Part model, mm, in its own coordinate system. A direction names the side the tool comes from. Give positions to 0.01 mm unless a question says otherwise; leave off trailing zeros. Write each loop counter-clockwise with the first axis right and the second up, starting at its lowest first coordinate (ties: lowest second). Pieces come first, ordered by that corner, then holes.
from build123d import *

# Parameters (mm, degrees)
SKETCH1_R           = 1.5
BOSS_EXTRUDE1_DEPTH = 2
SKETCH3_OUTSIDE_W   = 31.914
SKETCH3_OUTSIDE_H   = 31.796
SKETCH3_OUTSIDE_R   = 11.40725
CUT_EXTRUDE1_DEPTH  = 17.630863493
SKETCH4_R           = 2.5
CUT_EXTRUDE2_DEPTH  = 17.245136509
SKETCH5_R           = 2
BOSS_EXTRUDE2_DEPTH = 2
CUT_EXTRUDE3_DEPTH  = 35.968258573
CUT_EXTRUDE4_DEPTH  = 35.968258573
FILLET1_R           = 10


with BuildPart() as part:
    # Sketch1 → Boss-Extrude1 (new body)
    with BuildSketch(Plane(origin=(-1.354941904, 0, 0), x_dir=(0, 0, -1), z_dir=(1, 0, 0))):
        with BuildLine():
            ThreePointArc((-11.66138775, 0.780827758), (-10.210393031, 0.057188521), (-8.592596732, -0.051322118))
            ThreePointArc((-8.592596732, -0.051322118), (-8.545678016, -0.898186953), (-8.415498346, -1.736300708))
            ThreePointArc((-8.415498346, -1.736300708), (-9.975381284, -2.178798893), (-11.24421523, -3.188303642))
            ThreePointArc((-11.24421523, -3.188303642), (-11.115473034, -3.611636122), (-10.97079907, -4.029792056))
            ThreePointArc((-10.97079907, -4.029792056), (-9.350918841, -4.100696673), (-7.828853128, -3.541809038))
            ThreePointArc((-7.828853128, -3.541809038), (-7.441539788, -4.296375), (-6.981723166, -5.009081172))
            ThreePointArc((-6.981723166, -5.009081172), (-8.226766912, -6.047784929), (-8.975301827, -7.486094667))
            ThreePointArc((-8.975301827, -7.486094667), (-8.685505148, -7.820463962), (-8.383259564, -8.143624213))
            ThreePointArc((-8.383259564, -8.143624213), (-6.874585833, -7.549534157), (-5.711429695, -6.419884999))
            ThreePointArc((-5.711429695, -6.419884999), (-5.050691727, -6.951680778), (-4.340744624, -7.415745996))
            ThreePointArc((-4.340744624, -7.415745996), (-5.055669804, -8.871054007), (-5.154477201, -10.489471914))
            ThreePointArc((-5.154477201, -10.489471914), (-4.753734516, -10.677062536), (-4.34617832, -10.849349762))
            ThreePointArc((-4.34617832, -10.849349762), (-3.209574481, -9.692988601), (-2.606448181, -8.187904521))
            ThreePointArc((-2.606448181, -8.187904521), (-1.786533181, -8.404977796), (-0.949211902, -8.540160966))
            ThreePointArc((-0.949211902, -8.540160966), (-1.010401457, -10.160437258), (-0.442396639, -11.679124174))
            ThreePointArc((-0.442396639, -11.679124174), (0, -11.6875), (0.442396639, -11.679124174))
            ThreePointArc((0.442396639, -11.679124174), (1.010401457, -10.160437258), (0.949211902, -8.540160966))
            ThreePointArc((0.949211902, -8.540160966), (1.786533181, -8.404977796), (2.606448181, -8.187904521))
            ThreePointArc((2.606448181, -8.187904521), (3.209574481, -9.692988601), (4.34617832, -10.849349762))
            ThreePointArc((4.34617832, -10.849349762), (4.753734516, -10.677062536), (5.154477201, -10.489471914))
            ThreePointArc((5.154477201, -10.489471914), (5.055669804, -8.871054007), (4.340744624, -7.415745996))
            ThreePointArc((4.340744624, -7.415745996), (5.050691727, -6.951680778), (5.711429695, -6.419884999))
            ThreePointArc((5.711429695, -6.419884999), (6.874585833, -7.549534157), (8.383259564, -8.143624213))
            ThreePointArc((8.383259564, -8.143624213), (8.685505148, -7.820463962), (8.975301827, -7.486094667))
            ThreePointArc((8.975301827, -7.486094667), (8.226766912, -6.047784929), (6.981723166, -5.009081172))
            ThreePointArc((6.981723166, -5.009081172), (7.441539788, -4.296375), (7.828853128, -3.541809038))
            ThreePointArc((7.828853128, -3.541809038), (9.350918841, -4.100696673), (10.97079907, -4.029792056))
            ThreePointArc((10.97079907, -4.029792056), (11.115473034, -3.611636122), (11.24421523, -3.188303642))
            ThreePointArc((11.24421523, -3.188303642), (9.975381284, -2.178798893), (8.415498346, -1.736300708))
            ThreePointArc((8.415498346, -1.736300708), (8.545678016, -0.898186953), (8.592596732, -0.051322118))
            ThreePointArc((8.592596732, -0.051322118), (10.210393031, 0.057188521), (11.66138775, 0.780827758))
            ThreePointArc((11.66138775, 0.780827758), (11.623474652, 1.221676414), (11.568901669, 1.660774047))
            ThreePointArc((11.568901669, 1.660774047), (9.999161608, 2.066921265), (8.394157409, 1.836701922))
            ThreePointArc((8.394157409, 1.836701922), (8.17219088, 2.655305778), (7.8706023, 3.448038862))
            ThreePointArc((7.8706023, 3.448038862), (9.304397507, 4.205185299), (10.335616548, 5.456435359))
            ThreePointArc((10.335616548, 5.456435359), (10.121671907, 5.84375), (9.893219909, 6.222688815))
            ThreePointArc((9.893219909, 6.222688815), (8.29399605, 5.955251959), (6.921390398, 5.092122104))
            ThreePointArc((6.921390398, 5.092122104), (6.385657699, 5.749672018), (5.787709228, 6.351202599))
            ThreePointArc((5.787709228, 6.351202599), (6.789587127, 7.626067336), (7.222723349, 9.188575716))
            ThreePointArc((7.222723349, 9.188575716), (6.869740136, 9.455386122), (6.506910549, 9.708644156))
            ThreePointArc((6.506910549, 9.708644156), (5.154723227, 8.813865487), (4.251852108, 7.467068114))
            ThreePointArc((4.251852108, 7.467068114), (3.49498629, 7.849867731), (2.704068651, 8.156185707))
            ThreePointArc((2.704068651, 8.156185707), (3.100795451, 9.728333051), (2.860955666, 11.331927856))
            ThreePointArc((2.860955666, 11.331927856), (2.429967886, 11.432100084), (1.995497243, 11.515886722))
            ThreePointArc((1.995497243, 11.515886722), (1.124151929, 10.148481601), (0.847129962, 8.55089021))
            ThreePointArc((0.847129962, 8.55089021), (0, 8.59275), (-0.847129962, 8.55089021))
            ThreePointArc((-0.847129962, 8.55089021), (-1.124151929, 10.148481601), (-1.995497243, 11.515886722))
            ThreePointArc((-1.995497243, 11.515886722), (-2.429967886, 11.432100084), (-2.860955666, 11.331927856))
            ThreePointArc((-2.860955666, 11.331927856), (-3.100795451, 9.728333051), (-2.704068651, 8.156185707))
            ThreePointArc((-2.704068651, 8.156185707), (-3.49498629, 7.849867731), (-4.251852108, 7.467068114))
            ThreePointArc((-4.251852108, 7.467068114), (-5.154723227, 8.813865487), (-6.506910549, 9.708644156))
            ThreePointArc((-6.506910549, 9.708644156), (-6.869740136, 9.455386122), (-7.222723349, 9.188575716))
            ThreePointArc((-7.222723349, 9.188575716), (-6.789587127, 7.626067336), (-5.787709228, 6.351202599))
            ThreePointArc((-5.787709228, 6.351202599), (-6.385657699, 5.749672018), (-6.921390398, 5.092122104))
            ThreePointArc((-6.921390398, 5.092122104), (-8.29399605, 5.955251959), (-9.893219909, 6.222688815))
            ThreePointArc((-9.893219909, 6.222688815), (-10.121671907, 5.84375), (-10.335616548, 5.456435359))
            ThreePointArc((-10.335616548, 5.456435359), (-9.304397507, 4.205185299), (-7.8706023, 3.448038862))
            ThreePointArc((-7.8706023, 3.448038862), (-8.17219088, 2.655305778), (-8.394157409, 1.836701922))
            ThreePointArc((-8.394157409, 1.836701922), (-9.999161608, 2.066921265), (-11.568901669, 1.660774047))
            ThreePointArc((-11.568901669, 1.660774047), (-11.623474652, 1.221676414), (-11.66138775, 0.780827758))
        make_face()
        with Locations(Location((0, 0, 0), (0, 0, 180))):
            Circle(SKETCH1_R, mode=Mode.SUBTRACT)
    extrude(amount=-BOSS_EXTRUDE1_DEPTH)

    # Sketch3 outside → Cut-Extrude1 (cut, through all)
    with BuildSketch(Plane(origin=(-1.354941904, 0, 0), x_dir=(0, 0, -1), z_dir=(1, 0, 0))):
        with Locations((0, -0.086)):
            Rectangle(SKETCH3_OUTSIDE_W, SKETCH3_OUTSIDE_H)
        Circle(SKETCH3_OUTSIDE_R, mode=Mode.SUBTRACT)
    extrude(amount=-CUT_EXTRUDE1_DEPTH, mode=Mode.SUBTRACT)

    # Sketch4 → Cut-Extrude2 (cut, through all)
    with BuildSketch(Plane.ZY.offset(3.354941904)):
        Circle(SKETCH4_R)
    extrude(amount=-CUT_EXTRUDE2_DEPTH, mode=Mode.SUBTRACT)

    # Sketch5 → Boss-Extrude2 (add)
    with BuildSketch(Plane(origin=(-1.354941904, 0, 0), x_dir=(0, 0, -1), z_dir=(1, 0, 0))):
        with BuildLine():
            Line((-3, -30), (-3, -2.958198886))
            Line((-3, -2.958198886), (3, -2.958198886))
            Line((3, -2.958198886), (3, -30))
            ThreePointArc((3, -30), (0, -33), (-3, -30))
        make_face()
        with Locations((0, -30)):
            Circle(SKETCH5_R, mode=Mode.SUBTRACT)
    extrude(amount=-BOSS_EXTRUDE2_DEPTH)

    # Sketch6 → Cut-Extrude3 (cut, through all)
    with BuildSketch(Plane(origin=(-1.354941904, 0, 0), x_dir=(0, 0, -1), z_dir=(1, 0, 0))):
        with BuildLine():
            Line((3, -11.005696369), (3, -5.766281297))
            ThreePointArc((3, -5.766281297), (6.480220208, 0.506701151), (2.067265096, 6.162500712))
            Line((2.067265096, 6.162500712), (3.627970733, 10.81495173))
            ThreePointArc((3.627970733, 10.81495173), (11.4025291, -0.328150407), (3, -11.005696369))
        make_face()
    extrude(amount=-CUT_EXTRUDE3_DEPTH, mode=Mode.SUBTRACT)

    # Sketch7 → Cut-Extrude4 (cut, through all)
    with BuildSketch(Plane(origin=(-1.354941904, 0, 0), x_dir=(0, 0, -1), z_dir=(1, 0, 0))):
        with BuildLine():
            Line((-3, -11.005696369), (-3, -8.052040273))
            ThreePointArc((-3, -8.052040273), (-3.929768687, -7.641483536), (-4.804556181, -7.124015193))
            Line((-4.804556181, -7.124015193), (-6.378257659, -9.457440552))
            ThreePointArc((-6.378257659, -9.457440552), (-4.752599625, -10.370060239), (-3, -11.005696369))
        make_face()
    extrude(amount=-CUT_EXTRUDE4_DEPTH, mode=Mode.SUBTRACT)

    # Fillet1
    # the kernel refuses this fillet: 10 mm, written as the material it adds along each edge
    with BuildSketch(Plane(origin=(-1.354941904, -8.052040273, 3), x_dir=(0, -1, 0), z_dir=(-1, 0, 0))) as fillet1_piece_1:
        with BuildLine():
            CenterArc((5.214503978, 10), FILLET1_R, 226.79066028, 43.20933972)
            Line((-1.632155274, 2.711429695), (-1.769088459, 2.565658289))
            ThreePointArc((-1.769088459, 2.565658289), (-0.861521793, 1.328359568), (-0.187414746, -0.069826307))
            Line((-0.187414746, -0.069826307), (0, -0.2))
            Line((0, -0.2), (5.214503978, -0.2))
            Line((5.214503978, -0.2), (5.214503978, 0))
        make_face()
    extrude(amount=2)
    with BuildSketch(Plane(origin=(-1.354941904, 6.162500712, -2.067265096), x_dir=(0, 0.9480770325968022, -0.3180407839608656), z_dir=(-1, 0, 0))) as fillet1_piece_2:
        with BuildLine():
            CenterArc((7.819359493, 8.197923134), FILLET1_R, 209.791407991, 25.272600943)
            Line((-0.8590402, 3.229484871), (-1.032608194, 3.130116106))
            ThreePointArc((-1.032608194, 3.130116106), (-0.411709255, 1.619480105), (-0.2, 0))
            Line((-0.2, 0), (0, -0.2))
            ThreePointArc((0, -0.2), (1.046375, -0.2), (1.97821781, -0.163958463))
            Line((1.97821781, -0.163958463), (2.09275, 0))
        make_face()
    extrude(amount=2)
    with BuildSketch(Plane(origin=(-1.354941904, -5.766281297, -3), x_dir=(0, 0.6392655253408549, -0.7689860779693485), z_dir=(-1, 0, 0))) as fillet1_piece_3:
        with BuildLine():
            CenterArc((4.880340308, 9.772287101), FILLET1_R, 219.737073353, 38.012279544)
            Line((-2.809520471, 3.379631847), (-2.963317687, 3.251778742))
            Line((-2.963317687, 3.251778742), (-0.153797216, -0.127853105))
            Line((-0.153797216, -0.127853105), (0.042437742, -0.195445742))
            ThreePointArc((0.042437742, -0.195445742), (1.379226609, -0.051986615), (2.716015476, -0.195445742))
            Line((2.716015476, -0.195445742), (2.758453218, 0))
        make_face()
    extrude(amount=2)


solid = part.part
1) Saw through at A-A (z = 0). Write the cut outline in (x, y).
Check result:
outline: (-3.35, -33) - (-1.35, -33) - (-1.35, -32) - (-3.35, -32) - close; (-3.35, -28) - (-1.35, -28) - (-1.35, -2.5) - (-3.35, -2.5) - close; (-3.35, 2.5) - (-1.35, 2.5) - (-1.35, 8.59) - (-3.35, 8.59) - close
2) 3-axis set-ups, long thin cutter, end or side, ignore diameter. For faces 1 (the cylindrical face through (-2.37, -2.44, -0.54)), 2 (the cylindrical face through (-2.341, 6.089, -3.598)): which of +Z, -Z, +X, -X, +Y, -Y reach the whole face in a straight line?
Check result:
face 1: +X, -X
face 2: -Z, +X, -X
3) Flat gauge pins, fed straight in: P1, Ø2.5, axis at y = -30, z = 0, coming from the +X side; P2, Ø1, axis at x = -2, y = -16.5, coming from the -Z side; P3, Ø1, axis at x = -2.5, z = 4, coming from the +Y side. Where does each tip first touch, or does it go through?
Check result:
P1: passes through
P2: stops at z = -3
P3: stops at y = 7.97
4) Drill centre lines: L1, parallel to Y at x = -2.5, z = 0; L2, parallel to Y at x = -2.2, z = 9.5; L3, parallel to Z at x = -1.6, y = 9.5. Where is each one in solid material? Low to high.
Check result:
L1: y = -33 to -32, -28 to -2.5, 2.5 to 8.59
L2: y = -4.12 to -1.97, -0.07 to 2.06, 4.38 to 6.22
L3: z = -3.08 to -0.93, 0.93 to 3.08, 6.07 to 6.31
5) Saw through at C-C (y = -20.5). Write the cut outline in (x, z).
Check result:
outline: (-3.35, -3) - (-1.35, -3) - (-1.35, 3) - (-3.35, 3) - close
6) Saw through at B-B (x = -2.5). State how many separate pieces and enclosed holes the cut face has, and give its area (3 significant figures).
Check result:
separate pieces: 1
enclosed holes: 2
area: 350 mm2
7) Saw through at D-D (y = 3). Write the cut outline in (x, z).
Check result:
outline: (-3.35, -5.77) - (-1.35, -5.77) - (-1.35, 8.05) - (-3.35, 8.05) - close
